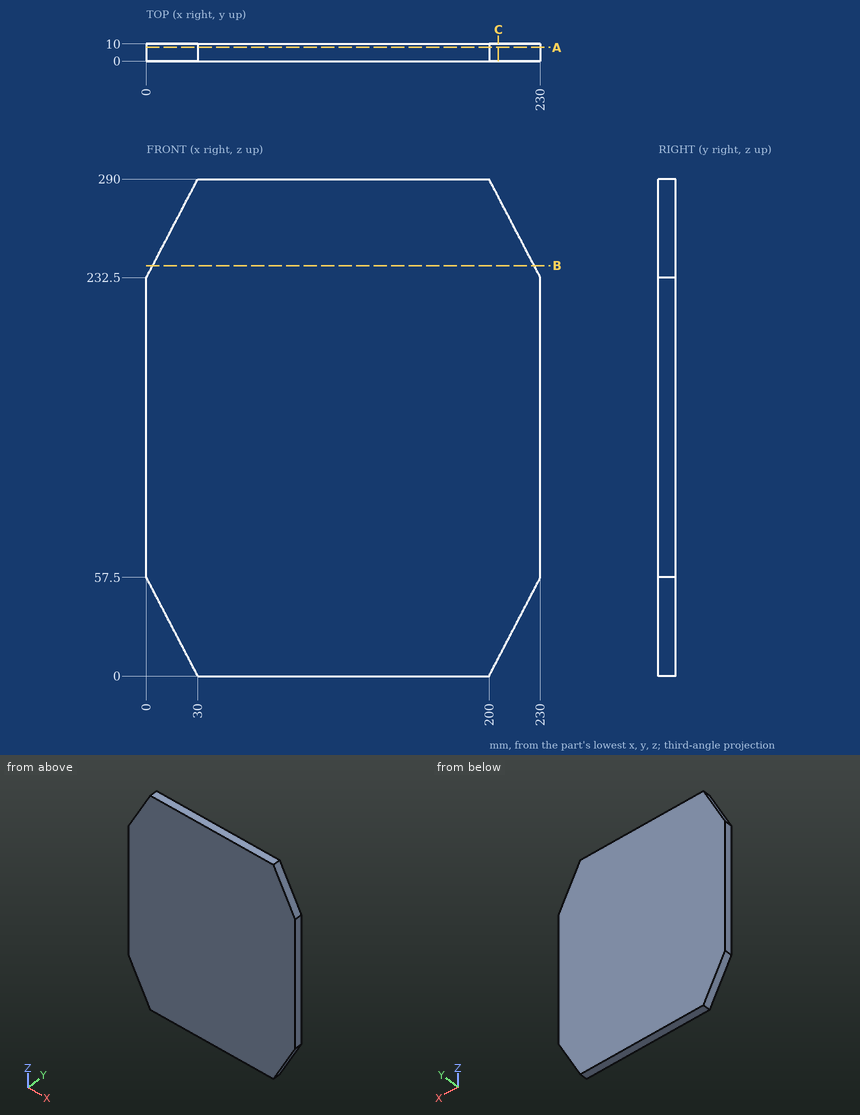
Source: three-view drawing plus pictorial views. Frame: mm from the lowest corner of the part. Coordinates: 2 decimals unless noted, no trailing zeros. Write each loop counter-clockwise with the first axis right and the second up, starting at its lowest first coordinate (ties: lowest second). Pieces come first, ordered by that corner, then holes. Notation, with made-up numbers: (69.25, -0.75) - (89.25, -0.75) arc R33 cw to (89.25, 27.25) - close; hole circle Ø10 at (61, -16). An arc over 180 degrees is marked (long way). Answer as a JSON object with one key per item and string values.
Q1. Material intervals for line 1 (X direction, y = 2.75, z = 39); line 2 (X direction, y = 7.5, z = 42); line 3 (Z direction, x = 12.5, y = 9.5), sorted ascending. Write a range as [from, to].
Ans:
{"line 1": "x = [9.65, 220.35]", "line 2": "x = [8.09, 221.91]", "line 3": "z = [33.54, 256.46]"}
Q2. Section query A-A, the plane y = 8. Output: boundary loops of the cut face in (x, z).
Ans:
{"outline": "(0, 57.5) - (30, 0) - (200, 0) - (230, 57.5) - (230, 232.5) - (200, 290) - (30, 290) - (0, 232.5) - close"}
Q3. Section query C-C, the plane x = 205.5. Output: boundary loops of the cut face in (y, z), plus the area to 3 significant figures.
Ans:
{"outline": "(0, 10.54) - (10, 10.54) - (10, 279.46) - (0, 279.46) - close", "area": "2,690 mm2"}
Q4. Section query B-B, the plane z = 239.5. Output: boundary loops of the cut face in (x, y), plus the area to 3 significant figures.
Ans:
{"outline": "(3.65, 0) - (226.35, 0) - (226.35, 10) - (3.65, 10) - close", "area": "2,230 mm2"}
